from build123d import *

# Parameters (mm, degrees)
SKETCH1_W           = 98
SKETCH1_H           = 15
BOSS_EXTRUDE1_DEPTH = 1
SKETCH2_W           = 1.052631579
SKETCH2_H           = 3.789473684
SKETCH2_W_2         = 2.526315789
SKETCH2_H_2         = 8
SKETCH2_W_3         = 2.315789474
SKETCH2_H_3         = 2.210526316
SKETCH2_W_4         = 6.105263158
SKETCH2_H_4         = 4
CUT_EXTRUDE1_DEPTH  = 10
SKETCH3_W           = 2.52631579
SKETCH3_H           = 0.5
SKETCH3_W_2         = 2.526315789
BOSS_EXTRUDE2_DEPTH = 1


with BuildPart() as part:
    # Sketch1 → Boss-Extrude1 (new body)
    with BuildSketch(Plane.XY):
        with Locations((0, 8.339183832)):
            Rectangle(SKETCH1_W, SKETCH1_H)
    extrude(amount=BOSS_EXTRUDE1_DEPTH)

    # Sketch2 → Cut-Extrude1 (cut)
    # profile 1 of 9: a face of its own
    with BuildSketch(Plane.XY.offset(1)):
        Polygon((-28.894736842, 4.339183832), (-28.894736842, 7.9181312), (-26.578947368, 7.9181312), (-26.578947368, 6.2931312), (-25.842105263, 7.2931312), (-25.842105263, 10.339183832), (-27.672697368, 10.339183832), (-27.672697368, 12.339183832), (-23.315789474, 12.339183832), (-23.315789474, 6.362210148), (-24.986842105, 4.339183832), align=None)
    # profile 2 of 9: a face of its own
    with BuildSketch(Plane.XY.offset(1)):
        Polygon((-22.263157895, 4.339183832), (-22.263157895, 10.870433832), (-20.503289474, 12.339183832), (-16.157894737, 12.339183832), (-16.157894737, 5.807933832), (-17.917763158, 4.339183832), align=None)
        with Locations((-19.210526316, 8.44444699)):
            Rectangle(SKETCH2_W, SKETCH2_H, mode=Mode.SUBTRACT)
    # profile 3 of 9: a face of its own
    with BuildSketch(Plane.XY.offset(1)):
        Polygon((-15.105263158, 4.339183832), (-15.105263158, 12.339183832), (-12.578947368, 12.339183832), (-12.578947368, 6.339183832), (-9.792763158, 6.339183832), (-9.792763158, 4.339183832), align=None)
    # profile 4 of 9: a face of its own
    with BuildSketch(Plane.XY.offset(1)):
        Polygon((-7.736842105, 4.339183832), (-7.736842105, 10.339183832), (-9.375, 10.339183832), (-9.375, 12.339183832), (-3.572368421, 12.339183832), (-3.572368421, 10.339183832), (-5.210526316, 10.339183832), (-5.210526316, 4.339183832), align=None)
    # profile 5 of 9: a face of its own
    with BuildSketch(Plane.XY.offset(1)):
        with Locations((-1.52631579, 8.339183832)):
            Rectangle(SKETCH2_W_2, SKETCH2_H_2)
    # profile 6 of 9: a face of its own
    with BuildSketch(Plane.XY.offset(1)):
        Polygon((4.368421053, 12.339183832), (6.894736842, 12.339183832), (6.894736842, 9.875368043), (5.371710526, 8.485565411), (6.894736842, 7.039841727), (6.894736842, 4.339183832), (4.368421053, 4.339183832), (4.368421053, 7.021749621), (3.315789474, 7.977341727), (3.315789474, 4.339183832), (0.789473684, 4.339183832), (0.789473684, 12.339183832), (3.315789474, 12.339183832), (3.315789474, 9.00694699), (4.368421053, 9.860565411), align=None)
    # profile 7 of 9: a face of its own
    with BuildSketch(Plane.XY.offset(1)):
        Polygon((18.052631579, 4.339183832), (11.947368421, 4.339183832), (11.947368421, 7.707604885), (13.496710526, 9.076025937), (15.526315789, 9.076025937), (15.526315789, 10.339183832), (11.947368421, 10.339183832), (11.947368421, 12.339183832), (18.052631579, 12.339183832), (18.052631579, 9.3556312), (16.526315789, 7.707604885), (14.473684211, 7.707604885), (14.473684211, 6.549710148), (18.052631579, 6.549710148), align=None)
    # profile 8 of 9: a face of its own
    with BuildSketch(Plane.XY.offset(1)):
        with Locations((20.263157895, 5.44444699)):
            Rectangle(SKETCH2_W_3, SKETCH2_H_3)
    # profile 9 of 9: a face of its own
    with BuildSketch(Plane.XY.offset(1)):
        with Locations((25.631578947, 8.339183832)):
            Rectangle(SKETCH2_W_4, SKETCH2_H_2)
        with Locations((25.631578948, 8.339183832)):
            Rectangle(SKETCH2_W, SKETCH2_H_4, mode=Mode.SUBTRACT)
    extrude(amount=-CUT_EXTRUDE1_DEPTH, mode=Mode.SUBTRACT)


with BuildPart() as cut_extrude1_piece_1:
    # of the separate pieces the step leaves, piece 1, a body of its own (cut_extrude1_pieces)
    add(part.part.solids().sort_by_distance((49, 15.839183832, 0))[0])



with BuildPart() as cut_extrude1_piece_2:
    # of the separate pieces the step leaves, piece 2, a body of its own (cut_extrude1_pieces)
    add(part.part.solids().sort_by_distance((26.157894737, 10.339183832, 0))[0])


with BuildPart() as cut_extrude1_piece_3:
    # of the separate pieces the step leaves, piece 3, a body of its own (cut_extrude1_pieces)
    add(part.part.solids().sort_by_distance((-18.684210526, 10.339183832, 0))[0])


with BuildPart() as cut_extrude1_piece_1_1:
    add(cut_extrude1_piece_1.part)

    add(cut_extrude1_piece_2.part)  # Boss-Extrude2 merges Cut-Extrude1 piece 2

    add(cut_extrude1_piece_3.part)  # Boss-Extrude2 merges Cut-Extrude1 piece 3
    # Sketch3 → Boss-Extrude2 (add)
    with BuildSketch(Plane.XY.offset(1)):
        with Locations((-21, 8.44444699)):
            Rectangle(SKETCH3_W, SKETCH3_H)
        with Locations((-17.421052632, 8.44444699)):
            Rectangle(SKETCH3_W_2, SKETCH3_H)
        with Locations((23.842105263, 8.339183832)):
            Rectangle(SKETCH3_W, SKETCH3_H)
        with Locations((27.421052632, 8.339183832)):
            Rectangle(SKETCH3_W_2, SKETCH3_H)
    extrude(amount=-BOSS_EXTRUDE2_DEPTH)


solid = cut_extrude1_piece_1_1.part
Part model, mm, in its own coordinate system. Coordinates: 2 decimals unless noted, no trailing zeros. One line per question, with ' | ' between items.
Q1. Slice it at A-A (z = 0.5). Count the separate pieces of the cut face and the enclosed holes in it, and give its area (3 significant figures).
A:
separate pieces: 1 | enclosed holes: 11 | area: 1,200 mm^2
Q2. Drill centre lines: line 1 (Y direction, x = -20, z = 0.1); line 2 (Y direction, x = 20.5, z = 0.6); line 3 (Y direction, x = -28.5, z = 0.75). Where is each one in solid material? Low to high.
A:
line 1: y = 0.84 to 4.34, 8.19 to 8.69, 12.34 to 15.84 | line 2: y = 0.84 to 4.34, 6.55 to 15.84 | line 3: y = 0.84 to 4.34, 7.92 to 15.84
Q3. Two-plate mould, pull along X, no slides. Class faces 1 (the face through (-1, 13, 1)), 2 (the face through (-24.14, 5.365, 0.507)), 3 (the face through (17.3, 8.543, 0.507)): +X half, -X half, draft (parallel to the pull), parting line (faces both ways), or undercut.
A:
face 1: draft | face 2: undercut | face 3: undercut
